Part print with two shaded views. Sizes in mm from the minimum x, y, z corner. A direction names the side the tool comes from. Round coordinates to 2 decimals unless told otherwise and drop trailing zeros. Order: outer loops, then holes, each group sorted by start corner. A loop starts at its lowest first (then second) coordinate and runs counter-clockwise, first axis right, second up. Notation, with made-up numbers: M 85.5,9.5 L 139.5,9.5 A21 cw 139.5,23.5 Z; hole C -16,18 d6. An arc over 180 degrees is marked long. Return JSON: item names as keys, results as strings. Group by question number.
Item 1: Which spindle directions (+Z, -Z, +X, -X, +Y, -Y) get a long thin tool onto all of the face, cutting with end or side? Do the marked faces 1 and 2. Say none if no direction does.
Item 2: Probe line 1 along X through (y, z) = (1.25, 21.5); line 2 along Z through (x, y) = (3, 0.85); line 3 along X through (y, z) = (2.7, 11). List the from-to ranges inside material, lowest first.
Item 3: Slice it at D-D on x = 20. Write the cut outline in (y, z).
Item 4: Slice it at A-A on z = 22. Write the cut outline in (x, y).
Item 5: Slice it at B-B on y = 0.7. Write the cut outline in (x, z).
Item 6: Slice it at C-C on z = 8. Write the cut outline in (x, y).
Item 7: Pull direction Z, two halves, no side cores. Call the marked faces 3, 4, 5 and 6: pulls with the +Z half, pulls with the -Z half, needs draft (parallel to the pull), parting line crosses it, or undercut.
Item 8: Pin check, flat tips, straight feed: pin 1 Ø1.5 at (y, z) = (2.5, 8.5) entering from -X; pin 2 Ø0.9 at (x, y) = (2.5, 1.5) entering from -Z; pin 3 Ø0.9 at (x, y) = (37, 2) entering from -Z. Stop position of each tip, or through.
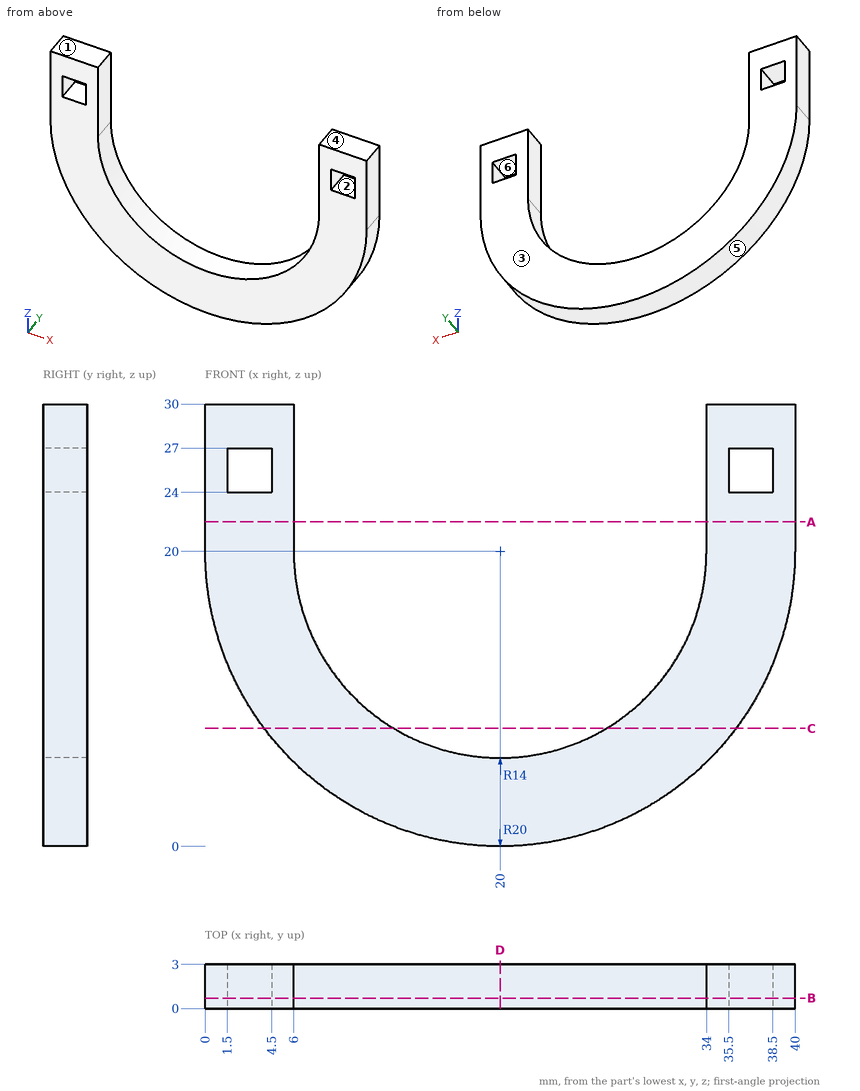
Output values:
{
 "1": {"face 1": "+Z, +X, -X, +Y, -Y", "face 2": "+Y, -Y"},
 "2": {"line 1": "0 to 6, 34 to 40", "line 2": "9.46 to 24, 27 to 30", "line 3": "2.14 to 9.28, 30.72 to 37.86"},
 "3": {"outline": "M 0,0 L 3,0 L 3,6 L 0,6 Z"},
 "4": {"outline": "M 0,0 L 6,0 L 6,3 L 0,3 Z; M 34,0 L 40,0 L 40,3 L 34,3 Z"},
 "5": {"outline": "M 0,20 A20 ccw 40,20 L 40,30 L 34,30 L 34,20 A14 cw 6,20 L 6,30 L 0,30 Z; hole M 1.5,24 L 4.5,24 L 4.5,27 L 1.5,27 Z; hole M 35.5,24 L 38.5,24 L 38.5,27 L 35.5,27 Z"},
 "6": {"outline": "M 4,0 L 12.79,0 L 12.79,3 L 4,3 Z; M 27.21,0 L 36,0 L 36,3 L 27.21,3 Z"},
 "7": {"face 3": "needs draft", "face 4": "pulls with the +Z half", "face 5": "pulls with the -Z half", "face 6": "undercut"},
 "8": {"pin 1": "x = 3.13", "pin 2": "z = 9.55", "pin 3": "z = 8.77"}
}
